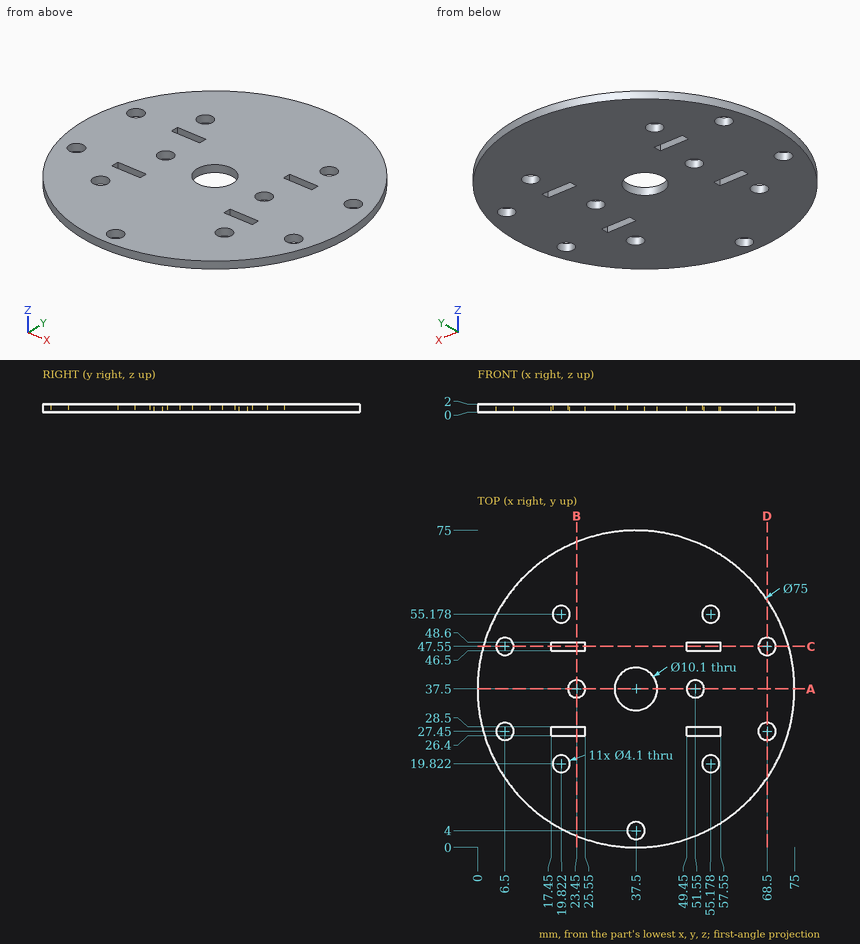
Job drawing, mm, ordinate dimensions from the low corner. One solid piece. Coordinates: 2 decimals unless noted, no trailing zeros. Order: outer loops, then holes, each group sorted by start corner. A loop starts at its lowest first (then second) coordinate and runs counter-clockwise, first axis right, second up. Notation, with made-up numbers: (85, 59) -> (130, 59) arc R9 ccw to (130, 64) -> close; hole circle Ø8 at (-8, 18.5). An arc over 180 degrees is marked (long way). Return JSON: item names as keys, results as strings. Group by question number.
Item 1: Saw through at D-D on x = 68.5. Write the cut outline in (y, z).
Item 2: Wall check: line 1 along Y through (x, z) = (68.5, 1.45); line 2 along Y through (x, z) = (37.5, 1.45); line 3 along Y through (x, z) = (50, 0.85) (1 decimal). Give the ranges that are in metal, low to high. Write a range as [from, to].
Item 3: Flat gauge pins, fed straight in: P1, Ø0.6, axis at x = 54, z = 0.5, coming from the +Y side; P2, Ø12, axis at x = 61, y = 15, coming from the -Z side; P3, Ø6, axis at x = 37.5, y = 37.5, coming from the -Z side; P4, Ø1, axis at x = 53.5, z = 1, coming from the +Y side. Where does each tip first touch, or does it go through?
Item 4: Saw through at C-C on y = 47.55. Write the cut outline in (x, z).
Item 5: Saw through at B-B on x = 23.45. Write the cut outline in (y, z).
Item 6: Saw through at A-A on y = 37.5. Write the cut outline in (x, z), then the cut area to 3 significant figures.
Values found:
{
 "1": {"outline": "(16.4, 0) -> (25.4, 0) -> (25.4, 2) -> (16.4, 2) -> close; (29.5, 0) -> (45.5, 0) -> (45.5, 2) -> (29.5, 2) -> close; (49.6, 0) -> (58.6, 0) -> (58.6, 2) -> (49.6, 2) -> close"},
 "2": {"line 1": "y = [16.4, 25.4], [29.5, 45.5], [49.6, 58.6]", "line 2": "y = [0, 1.95], [6.05, 32.45], [42.55, 75]", "line 3": "y = [2.1, 26.4], [28.5, 36.2], [38.8, 46.5], [48.6, 72.9]"},
 "3": {"P1": "stops at y = 71.32", "P2": "stops at z = 0", "P3": "passes through", "P4": "stops at y = 71.65"},
 "4": {"outline": "(1.37, 0) -> (4.45, 0) -> (4.45, 2) -> (1.37, 2) -> close; (8.55, 0) -> (17.45, 0) -> (17.45, 2) -> (8.55, 2) -> close; (25.55, 0) -> (49.45, 0) -> (49.45, 2) -> (25.55, 2) -> close; (57.55, 0) -> (66.45, 0) -> (66.45, 2) -> (57.55, 2) -> close; (70.55, 0) -> (73.63, 0) -> (73.63, 2) -> (70.55, 2) -> close"},
 "5": {"outline": "(2.73, 0) -> (26.4, 0) -> (26.4, 2) -> (2.73, 2) -> close; (28.5, 0) -> (35.45, 0) -> (35.45, 2) -> (28.5, 2) -> close; (39.55, 0) -> (46.5, 0) -> (46.5, 2) -> (39.55, 2) -> close; (48.6, 0) -> (72.27, 0) -> (72.27, 2) -> (48.6, 2) -> close"},
 "6": {"outline": "(0, 0) -> (21.4, 0) -> (21.4, 2) -> (0, 2) -> close; (25.5, 0) -> (32.45, 0) -> (32.45, 2) -> (25.5, 2) -> close; (42.55, 0) -> (49.5, 0) -> (49.5, 2) -> (42.55, 2) -> close; (53.6, 0) -> (75, 0) -> (75, 2) -> (53.6, 2) -> close", "area": "113 mm2"}
}
